Study the drawing (mm; zero at the part's minimum x, y, z) and answer. Give positions to 0.01 mm unless a question says otherwise; leave off trailing zeros. Put each result on its own line as item: value.
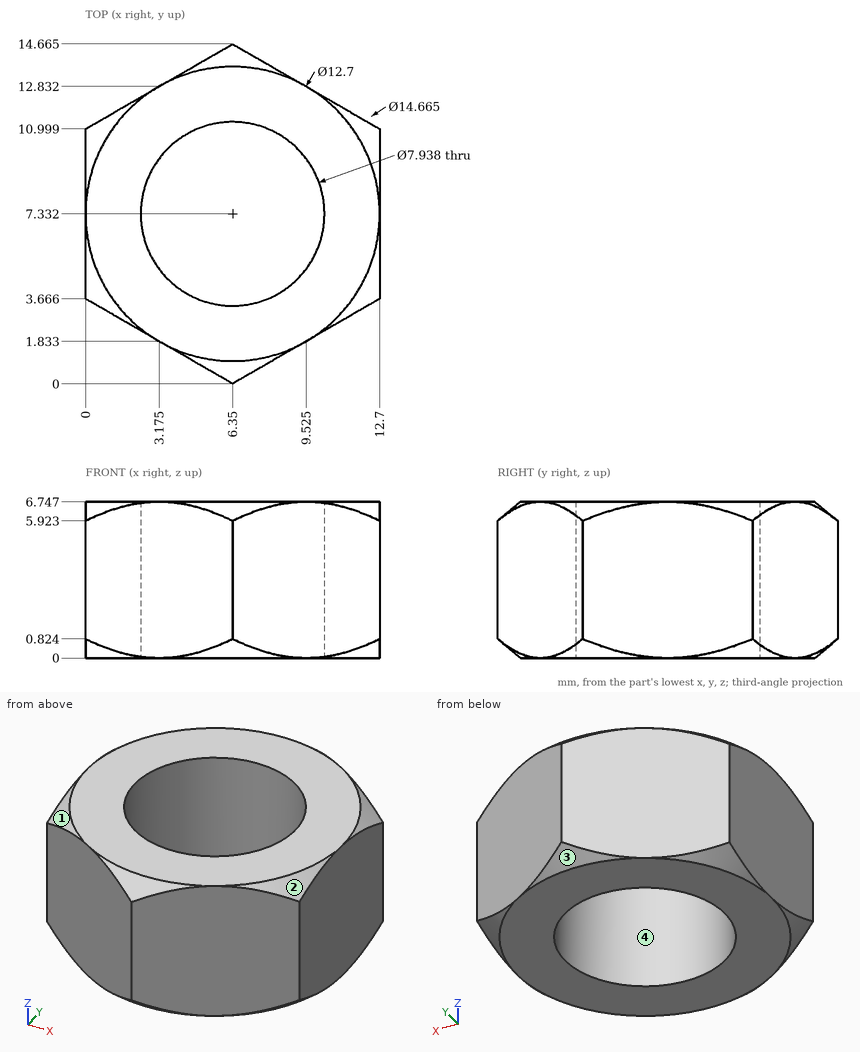
(1) Determine the mould class of the marked faces 1, 2, 3 and 4 for opening direction X: pulls with the +X half, pulls with the -X half, needs draft (parallel to the pull), parting line crosses it, or undercut.
Geometry check:
face 1: pulls with the -X half
face 2: pulls with the +X half
face 3: parting line crosses it
face 4: undercut
(2) Given pin 1 (4 mm diameter, centred on x = 9, z = 2.5, fed in from +Y); pin 2 (2 mm diameter, centred on x = 4.5, z = 1, fed in from -Y); pin 3 (1.5 mm diameter, centred on x = 5.5, z = 2, fed in from -Y), each flat-ended and moving along its own axis, determine where each tip first touches the part or whether it passes through.
Geometry check:
pin 1: stops at y = 14.29
pin 2: stops at y = 0.49
pin 3: stops at y = 0.06
(3) Straight lines are drawn through the part: line 1 (Y direction, x = 6, z = 1.75) (1 decimal); line 2 (X direction, y = 7.75, z = 6); line 3 (X direction, y = 10.5, z = 4). For each, find the intervals that lie inside material, in ascending order.
Geometry check:
line 1: y = 0.2 to 3.4, 11.3 to 14.5
line 2: x = 0 to 2.4, 10.3 to 12.7
line 3: x = 0 to 3.96, 8.74 to 12.7
